```python
from build123d import *

# Parameters (mm, degrees)
BOSS_EXTRUDE1_DEPTH                                 = 10
CSK_FOR_M3_COUNTERSUNK_FLAT_HEAD_SCREW1_D           = 3.4
CSK_FOR_M3_COUNTERSUNK_FLAT_HEAD_SCREW1_CSINK_D     = 6.3
CSK_FOR_M3_COUNTERSUNK_FLAT_HEAD_SCREW1_CSINK_ANGLE = 90
SKETCH4_W                                           = 12
SKETCH4_H                                           = 24
CUT_EXTRUDE1_DEPTH                                  = 10
SKETCH6_W                                           = 32
SKETCH6_H                                           = 7
BOSS_EXTRUDE3_DEPTH                                 = 10
SKETCH7_W                                           = 8
SKETCH7_H                                           = 42
BOSS_EXTRUDE4_DEPTH                                 = 47
SKETCH8_R                                           = 11.25
CUT_EXTRUDE2_DEPTH                                  = 47
CSK_FOR_M3_COUNTERSUNK_FLAT_HEAD_SCREW2_D           = 3.4
CSK_FOR_M3_COUNTERSUNK_FLAT_HEAD_SCREW2_CSINK_D     = 6.3
CSK_FOR_M3_COUNTERSUNK_FLAT_HEAD_SCREW2_CSINK_ANGLE = 90
FILLET1_R                                           = 8
FILLET2_R                                           = 1.5
FILLET3_R                                           = 3
FILLET4_R                                           = 2


with BuildPart() as part:
    # Sketch1 → Boss-Extrude1 (new body)
    with BuildSketch(Plane(origin=(0, 0, 0), x_dir=(0, 0, -1), z_dir=(1, 0, 0))):
        Polygon((0, 0), (-98.5, 0), (-98.5, 35), (0, 35), (5, 35), (5, 30), (0, 30), align=None)
    extrude(amount=BOSS_EXTRUDE1_DEPTH)

    # CSK for M3 Countersunk Flat Head Screw1 (through all)
    with Locations(Plane(origin=(0, 16, 8.5), x_dir=(0, 0, -1), z_dir=(-1, 0, 0))):
        with Locations((0, 0), (-60, -14), (-60, 11), (-80, 0)):
            CounterSinkHole(CSK_FOR_M3_COUNTERSUNK_FLAT_HEAD_SCREW1_D / 2, CSK_FOR_M3_COUNTERSUNK_FLAT_HEAD_SCREW1_CSINK_D / 2, counter_sink_angle=CSK_FOR_M3_COUNTERSUNK_FLAT_HEAD_SCREW1_CSINK_ANGLE)

    # Sketch4 → Cut-Extrude1 (cut)
    with BuildSketch(Plane.ZY):
        with Locations((24, 15)):
            Rectangle(SKETCH4_W, SKETCH4_H)
    extrude(amount=-CUT_EXTRUDE1_DEPTH, mode=Mode.SUBTRACT)

    # Sketch6 → Boss-Extrude3 (add)
    with BuildSketch(Plane.ZY):
        with Locations((34, -3.5)):
            Rectangle(SKETCH6_W, SKETCH6_H)
    extrude(amount=-BOSS_EXTRUDE3_DEPTH)

    # Sketch7 → Boss-Extrude4 (add)
    with BuildSketch(Plane.ZY):
        with Locations((34, 14)):
            Rectangle(SKETCH7_W, SKETCH7_H)
    extrude(amount=BOSS_EXTRUDE4_DEPTH)

    # Sketch8 → Cut-Extrude2 (cut)
    with BuildSketch(Plane(origin=(0, 0, 30), x_dir=(-1, 0, 0), z_dir=(0, 0, -1))):
        with Locations(Location((25, 13, 0), (0, 0, 90))):
            Circle(SKETCH8_R)
    extrude(amount=-CUT_EXTRUDE2_DEPTH, mode=Mode.SUBTRACT)

    # CSK for M3 Countersunk Flat Head Screw2 (through all)
    with Locations(Plane(origin=(-9.5, 28.5, 30), x_dir=(0, -1, 0), z_dir=(0, 0, -1))):
        with Locations((0, 0), (0, 31), (31, 31), (31, 0)):
            CounterSinkHole(CSK_FOR_M3_COUNTERSUNK_FLAT_HEAD_SCREW2_D / 2, CSK_FOR_M3_COUNTERSUNK_FLAT_HEAD_SCREW2_CSINK_D / 2, counter_sink_angle=CSK_FOR_M3_COUNTERSUNK_FLAT_HEAD_SCREW2_CSINK_ANGLE)

    # Fillet1
    fillet1_edges = [part.edges().sort_by_distance(p)[0] for p in [
        (5, 35, 98.5),
    ]]
    fillet(fillet1_edges, radius=FILLET1_R)

    # Fillet2
    fillet2_edges = [part.edges().sort_by_distance(p)[0] for p in [
        (5, -7, 18),
        (5, 0, 18),
        (5, 0, 50),
        (5, -7, 50),
    ]]
    fillet(fillet2_edges, radius=FILLET2_R)

    # Fillet3
    fillet3_edges = [part.edges().sort_by_distance(p)[0] for p in [
        (-47, -7, 34),
        (-47, 35, 34),
    ]]
    fillet(fillet3_edges, radius=FILLET3_R)

    # Fillet4
    fillet4_edges = [part.edges().sort_by_distance(p)[0] for p in [
        (0, -2, 30),
        (0, 31, 30),
        (0, 14, 38),
    ]]
    fillet(fillet4_edges, radius=FILLET4_R)


solid = part.part
```
Geometry check sheet. Reference: the model listing, model coordinates, mm. A direction names the side the tool comes from. Round coordinates to 2 decimals unless told otherwise and drop trailing zeros. Loops run counter-clockwise (first coordinate to the right, second up) from the corner with the lowest first, then second, coordinate; pieces in that order, holes last. Notation, with made-up numbers: M -37,68 L -22,68 A17 cw -22,79 Z; hole C -25,41.25 d4. An arc over 180 degrees is marked long. Return JSON: item names as keys, results as strings. Group by question number.
(1) Section check D-D, the plane y = 16. Enter the section's corners in (x, z), and give its area (3 significant figures).
(2) Section check C-C, the plane z = 35. Enter the section's corners in (x, y).
(3) Section check B-B, the plane x = -40.5. Enter the section's corners in (y, z).
(4) Set-up check for faces 4 (the face through (5, 27, 24)), 5 (the face through (-12, 14, 30)), 6 (the face through (5, 0, 8)), 7 (the face through (0, 14, 69)), 8 (the face through (5, 0, 75)): record each of +Z, -Z, +X, -X, +Y, -Y from which the full face is reachable in a straight line by a thin tool's end or side.
(5) Mould release check, pull along Z, two halves, no side actions. Record for faces 1 (the face through (5, 3, 24)), 2 (the face through (5, 30, -3)), 3 (the face through (-0.6, -1.93, 29.43)): pulls with the +Z half, pulls with the -Z half, needs draft (parallel to the pull), parting line crosses it, or undercut.
(6) Section check A-A, the plane z = 23.5. Enter the section's corners in (x, y).
(7) Go/stop test with flat-tipped pins: pin 1 (12 mm diameter, centred on x = -2.5, y = 14, fed in from -Z); pin 2 (5 mm diameter, centred on x = 7.5, z = 84, fed in from -Y); pin 3 (1.5 mm diameter, centred on x = 6.5, z = -2.5, fed in from -Y). Record where each tip stops, or that it passes through.
(8) Scan lines: line 1 along Y through (x, z) = (-9.5, 36.75); line 2 along X through (y, z) = (28.5, 36.5); line 3 along Z through (x, y) = (5, 5). Record each from-to range of solid material in increasing order. Write a range as [from, to].
Data:
{
 "1": {"outline": "M -47,30 L -35.84,30 L -35.84,38 L -47,38 Z; M -14.16,30 L 10,30 L 10,86.8 L 1.45,86.8 L 0,85.35 L 0,40 A2 cw -2,38 L -14.16,38 Z; M 0,0 L 10,0 L 10,6.8 L 1.45,6.8 L 0,5.35 Z; M 0,11.65 L 1.45,10.2 L 10,10.2 L 10,18 L 0,18 Z; M 0,91.65 L 1.45,90.2 L 10,90.2 L 10,98.5 L 0,98.5 Z", "area": "996 mm²"},
 "2": {"outline": "M -47,-4 A3 ccw -44,-7 L 10,-7 L 10,35 L -44,35 A3 ccw -47,32 Z; hole C -40.5,-2.5 d3.4; hole C -40.5,28.5 d3.4; hole C -25,13 d22.5; hole C -9.5,-2.5 d3.4; hole C -9.5,28.5 d3.4"},
 "3": {"outline": "M -7,30 L -5.65,30 L -4.2,31.45 L -4.2,38 L -7,38 Z; M -0.8,31.45 L 0.65,30 L 25.35,30 L 26.8,31.45 L 26.8,38 L -0.8,38 Z; M 30.2,31.45 L 31.65,30 L 35,30 L 35,38 L 30.2,38 Z"},
 "4": {"face 4": "+X, -X", "face 5": "-X", "face 6": "-Z, +X, -X, -Y", "face 7": "+Z, -X, +Y, -Y", "face 8": "+Z, +X, -X, -Y"},
 "5": {"face 1": "undercut", "face 2": "needs draft", "face 3": "pulls with the -Z half"},
 "6": {"outline": "M 0,-7 L 10,-7 L 10,3 L 0,3 Z; M 0,27 L 10,27 L 10,35 L 0,35 Z"},
 "7": {"pin 1": "z = 0", "pin 2": "y = 0", "pin 3": "y = 30"},
 "8": {"line 1": "[-7, -4.2], [-0.8, 26.8], [30.2, 35]", "line 2": "[-47, -42.2], [-38.8, -11.2], [-7.8, 10]", "line 3": "[0, 18], [30, 66.8], [70.2, 98.5]"}
}
